Could you check a few things on this model? Use its own coordinates, in mm. Round coordinates to 2 decimals unless told otherwise and drop trailing zeros. Loops run counter-clockwise (first coordinate to the right, second up) from the corner with the lowest first, then second, coordinate; pieces in that order, holes last. Notation, with made-up numbers: M -32.75,88.5 L 2.25,88.5 A28 ccw 2.25,122.5 Z; hole C -2.5,-20 d10. An arc over 180 degrees is marked long. Return JSON: item names as keys, results as strings. Group by question number.
```python
from build123d import *

# Parameters (mm, degrees)
SKETCH1_R               = 2.875
BOSS_EXTRUDE1_DEPTH     = 10
SKETCH2_R               = 1.625
CUT_EXTRUDE1_DEPTH      = 6
CUT_EXTRUDE1_DEPTH_BACK = 15.5


with BuildPart() as part:
    # Sketch1 → Boss-Extrude1 (new body)
    with BuildSketch(Plane.XY):
        with BuildLine():
            Line((0, -5), (-9.5, -5))
            ThreePointArc((-9.5, -5), (-14.5, 0), (-9.5, 5))
            Line((-9.5, 5), (0, 5))
            ThreePointArc((0, 5), (5, 0), (0, -5))
        make_face()
        Circle(SKETCH1_R, mode=Mode.SUBTRACT)
        with Locations((-9.5, 0)):
            Circle(SKETCH1_R, mode=Mode.SUBTRACT)
    extrude(amount=BOSS_EXTRUDE1_DEPTH)

    # Sketch2 → Cut-Extrude1 (cut, two sides)
    with BuildSketch(Plane(origin=(0, 0, 0), x_dir=(0, 0, -1), z_dir=(1, 0, 0))) as cut_extrude1_sk:
        with Locations((-5, 0)):
            Circle(SKETCH2_R)
    extrude(amount=CUT_EXTRUDE1_DEPTH, mode=Mode.SUBTRACT)
    extrude(cut_extrude1_sk.sketch, amount=-CUT_EXTRUDE1_DEPTH_BACK, mode=Mode.SUBTRACT)


solid = part.part
```
1. If we section it at A-A, the plane z = 2: Please give me the cut outline in (x, y) (3 decimals), then the cut area to 3 significant figures.
2. If we section it at D-D, the plane z = 5: Please give me the cut outline in (x, y) (3 decimals).
3. We'd pull the mould along X, two halves only. Please class faces 1 (the face through (-11.62, 1.94, 4.93)), 2 (the face through (-13.17, -0.99, 6.29)), 3 (the face through (-2.12, 1.94, 4.93)), 4 (the face through (-14.16, -1.81, 4.93)): +X half, -X half, draft (parallel to the pull), parting line (faces both ways), or undercut.
4. I need wall thicknesses on probe 1 along X at (y, z) = (0, 6.75) (3 decimals); probe 2 along Y at (x, z) = (-9.5, 4.25) (3 decimals); probe 3 along Y at (x, z) = (-4.05, 5) (3 decimals). Which ranges of each line are inside material? Lowest first, please.
5. If we section it at B-B, the plane x = -11.5: Please give me the cut outline in (y, z).
6. I'm going to push flat-ended pins straight in: pin 1 Ø6 at (y, z) = (-3.5, 6) entering from -X; pin 2 Ø1 at (x, y) = (-11.5, 1) entering from +Z; pin 3 Ø2 at (y, z) = (-4, 1.5) entering from +X. Where does each tip first touch, or does it pass through?
7. If we section it at C-C, the plane y = 0: Please give me the cut outline in (x, z) (3 decimals).
Geometry results:
{
 "1": {"outline": "M -9.5,-5 L 0,-5 A5 ccw 0,5 L -9.5,5 A5 ccw Z; hole C -9.5,0 d5.75; hole C 0,0 d5.75", "area": "122 mm^2"},
 "2": {"outline": "M -14.229,-1.625 A5 ccw -9.5,-5 L 0,-5 A5 ccw 4.729,-1.625 L 2.372,-1.625 A2.875 cw -2.372,-1.625 L -7.128,-1.625 A2.875 cw -11.872,-1.625 Z; M -14.229,1.625 L -11.872,1.625 A2.875 cw -7.128,1.625 L -2.372,1.625 A2.875 cw 2.372,1.625 L 4.729,1.625 A5 ccw 0,5 L -9.5,5 A5 ccw Z"},
 "3": {"face 1": "undercut", "face 2": "draft", "face 3": "undercut", "face 4": "-X half"},
 "4": {"probe 1": "-14.5 to -12.375, -6.625 to -2.875, 2.875 to 5", "probe 2": "-5 to -2.875, 2.875 to 5", "probe 3": "-5 to -1.625, 1.625 to 5"},
 "5": {"outline": "M -4.58,0 L -2.07,0 L -2.07,10 L -4.58,10 Z; M 2.07,0 L 4.58,0 L 4.58,10 L 2.07,10 Z"},
 "6": {"pin 1": "x = -14.47", "pin 2": "through", "pin 3": "x = 4"},
 "7": {"outline": "M -14.5,0 L -12.375,0 L -12.375,3.375 L -14.5,3.375 Z; M -14.5,6.625 L -12.375,6.625 L -12.375,10 L -14.5,10 Z; M -6.625,0 L -2.875,0 L -2.875,3.375 L -6.625,3.375 Z; M -6.625,6.625 L -2.875,6.625 L -2.875,10 L -6.625,10 Z; M 2.875,0 L 5,0 L 5,3.375 L 2.875,3.375 Z; M 2.875,6.625 L 5,6.625 L 5,10 L 2.875,10 Z"}
}
